from build123d import *

# Parameters (mm, degrees)
SKETCH1_R      = 11
EXTRUDE1_DEPTH = 2
SKETCH2_R      = 5
EXTRUDE2_DEPTH = 8
SKETCH3_R      = 1.5
EXTRUDE5_DEPTH = 19.493242009
SKETCH4_R      = 1.5
EXTRUDE6_DEPTH = 8


with BuildPart() as part:
    # Sketch1 → Extrude1 (new body)
    with BuildSketch(Plane.XY):
        Circle(SKETCH1_R)
    extrude(amount=EXTRUDE1_DEPTH)

    # Sketch2 → Extrude2 (add)
    with BuildSketch(Plane.XY.offset(2)):
        Circle(SKETCH2_R)
    extrude(amount=EXTRUDE2_DEPTH)

    # Sketch3 → Extrude5 (cut, through all)
    with BuildSketch(Plane.XY):
        Circle(SKETCH3_R)
    extrude(amount=EXTRUDE5_DEPTH, mode=Mode.SUBTRACT)

    # Sketch4 → Extrude6 (cut)
    with BuildSketch(Plane(origin=(0, 0, 0), x_dir=(-1, 0, 0), z_dir=(0, 0, -1))):
        with Locations((8, 0)):
            Circle(SKETCH4_R)
        with Locations((0, -8)):
            Circle(SKETCH4_R)
        with Locations((-8, 0)):
            Circle(SKETCH4_R)
        with Locations((0, 8)):
            Circle(SKETCH4_R)
    extrude(amount=-EXTRUDE6_DEPTH, mode=Mode.SUBTRACT)


solid = part.part
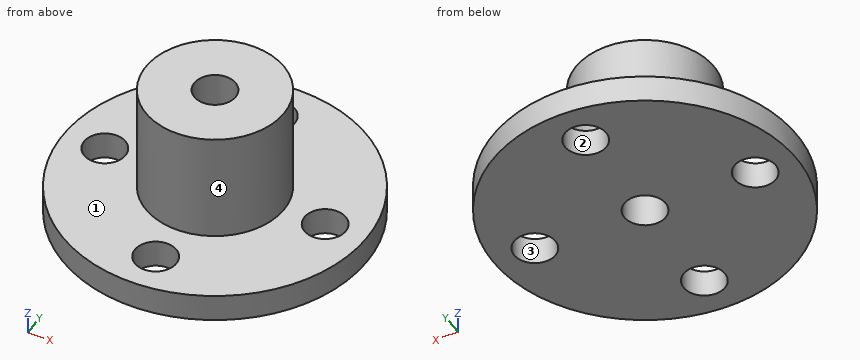
Geometry check sheet. Reference: the model listing, model coordinates, mm. Face numbers are marked on the shaded views. Give positions to 0.01 mm unless a question says otherwise; leave off trailing zeros. Write each loop counter-clockwise with the first axis right and the second up, starting at its lowest first coordinate (ties: lowest second). Pieces come first, ordered by that corner, then holes.
1) Release check for a two-part mould opening along X. For the marked faces 1, 2, 3 and 4 record: released by +X, released by -X, zero draft, split by the parting line, or undercut.
Values follow:
face 1: zero draft
face 2: undercut
face 3: undercut
face 4: split by the parting line
2) Thickness scan on line 1 (Y direction, x = 0, z = 1.65); line 2 (Z direction, x = -7.25, y = -4); line 3 (Y direction, x = -8, z = 1.25). Record the ranges inside material, lowest first.
Values follow:
line 1: y = -11 to -9.5, -6.5 to -1.5, 1.5 to 6.5, 9.5 to 11
line 2: z = 0 to 2
line 3: y = -7.55 to -1.5, 1.5 to 7.55
3) Go/stop test with flat-tipped pins: pin 1 Ø2.5 at (x, y) = (0, 0) entering from -Z (3 decimals); pin 2 Ø3 at (x, y) = (-6.5, 5.5) entering from +Z; pin 3 Ø2 at (y, z) = (-2, 6.5) entering from -X; pin 4 Ø4 at (y, z) = (0.5, 6) entering from +X. Record where each tip stops, or that it passes through.
Values follow:
pin 1: passes through
pin 2: stops at z = 2
pin 3: stops at x = -4.9
pin 4: stops at x = 5
4) Cross-section at D-D (x = -8). Record the boundary of the cut face in (y, z), plus the area to 3 significant figures.
Values follow:
outline: (-7.55, 0) - (-1.5, 0) - (-1.5, 2) - (-7.55, 2) - close; (1.5, 0) - (7.55, 0) - (7.55, 2) - (1.5, 2) - close
area: 24.2 mm2
5) Cross-section at A-A (y = 0). Record the boundary of the cut face in (x, z), plus the area to 3 significant figures.
Values follow:
outline: (-11, 0) - (-9.5, 0) - (-9.5, 2) - (-11, 2) - close; (-6.5, 0) - (-1.5, 0) - (-1.5, 10) - (-5, 10) - (-5, 2) - (-6.5, 2) - close; (1.5, 0) - (6.5, 0) - (6.5, 2) - (5, 2) - (5, 10) - (1.5, 10) - close; (9.5, 0) - (11, 0) - (11, 2) - (9.5, 2) - close
area: 82.0 mm2
6) Cross-section at C-C (y = -7). Record the boundary of the cut face in (x, z).
Values follow:
outline: (-8.49, 0) - (-1.12, 0) - (-1.12, 2) - (-8.49, 2) - close; (1.12, 0) - (8.49, 0) - (8.49, 2) - (1.12, 2) - close
